from build123d import *

# Parameters (mm, degrees)
F1_DEPTH = 25.4
F2_R     = 9.525
F3_DEPTH = 6.35
F4_R     = 15.875
F5_DEPTH = 6.35
F6_R     = 9.525
F7_DEPTH = 76.2
F8_DEPTH = 6.35


with BuildPart() as f1:
    # F0 (on Top) → F1 (new body, symmetric)
    with BuildSketch(Plane.XY):
        with BuildLine():
            ThreePointArc((0, -19.05), (13.470384, -13.470384), (19.05, 0))
            ThreePointArc((19.05, 0), (13.470384, 13.470384), (0, 19.05))
            ThreePointArc((0, 19.05), (-19.05, 0), (0, -19.05))
        make_face()
    extrude(amount=F1_DEPTH, both=True)

    # F2 (on face) → F3 (cut)
    with BuildSketch(Plane.XY.offset(12.7)):
        Circle(F2_R)
    extrude(amount=-F3_DEPTH, mode=Mode.SUBTRACT)

    # F4 (on face) → F5 (cut)
    with BuildSketch(Plane.XY.offset(19.05)):
        Circle(F4_R)
    extrude(amount=-F5_DEPTH, mode=Mode.SUBTRACT)

    # F6 (on face) → F7 (cut)
    with BuildSketch(Plane.XY.offset(25.4)):
        Circle(F6_R)
    extrude(amount=-F7_DEPTH, mode=Mode.SUBTRACT)

    # F0 (on Top) → F8 (join, symmetric)
    with BuildSketch(Plane.XY):
        with BuildLine():
            ThreePointArc((0, -19.05), (-19.05, 0), (0, 19.05))
            Line((0, 19.05), (-38.1, 19.05))
            Line((-38.1, 19.05), (-38.1, -19.05))
            Line((-38.1, -19.05), (0, -19.05))
        make_face()
        with BuildLine():
            ThreePointArc((0, 19.05), (13.470384, 13.470384), (19.05, 0))
            ThreePointArc((19.05, 0), (13.470384, -13.470384), (0, -19.05))
            Line((0, -19.05), (38.1, -19.05))
            Line((38.1, -19.05), (38.1, 19.05))
            Line((38.1, 19.05), (0, 19.05))
        make_face()
    extrude(amount=F8_DEPTH, both=True)


solid = f1.part
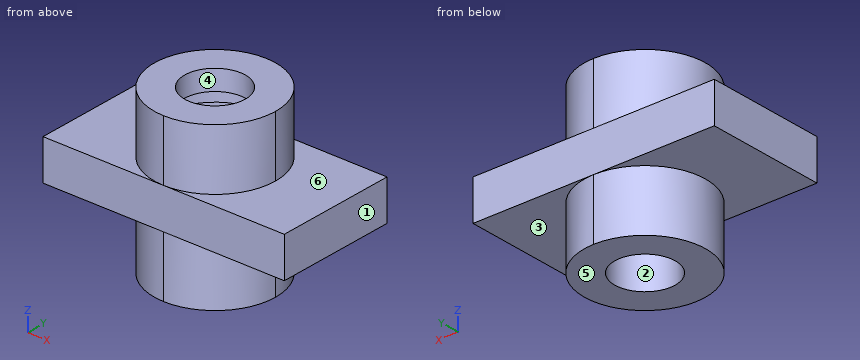
Can you work these out from the model? Positions are in its coordinate system, mm. Face numbers are marked on the shaded views. A direction names the side the tool comes from. Coordinates: 2 decimals unless noted, no trailing zeros. Order: outer loops, then holes, each group sorted by start corner. A loop starts at its lowest first (then second) coordinate and runs counter-clockwise, first axis right, second up. Notation, with made-up numbers: M 68.25,84.25 L 81.25,84.25 A29 cw 81.25,114.25 Z; hole C 14.5,-23 d7. An arc over 180 degrees is marked long. Write item = value, one per line.
(1) Suppose I cut it at C-C on x = -18. Please give me the cut outline in (y, z), plus the area to 3 significant figures.
Results are:
outline = M -19.05,-6.35 L -6.24,-6.35 L -6.24,-25.4 L 6.24,-25.4 L 6.24,-6.35 L 19.05,-6.35 L 19.05,6.35 L 6.24,6.35 L 6.24,25.4 L -6.24,25.4 L -6.24,6.35 L -19.05,6.35 Z
area = 959 mm2
(2) Suppose I cut it at A-A on y = 2.5. Please give me the cut outline in (x, z), plus the area to 3 significant figures.
Results are:
outline = M -38.1,-6.35 L -18.89,-6.35 L -18.89,-25.4 L -9.19,-25.4 L -9.19,12.7 L -15.68,12.7 L -15.68,19.05 L -9.19,19.05 L -9.19,25.4 L -18.89,25.4 L -18.89,6.35 L -38.1,6.35 Z; M 9.19,-25.4 L 18.89,-25.4 L 18.89,-6.35 L 38.1,-6.35 L 38.1,6.35 L 18.89,6.35 L 18.89,25.4 L 9.19,25.4 L 9.19,19.05 L 15.68,19.05 L 15.68,12.7 L 9.19,12.7 Z
area = 1,390 mm2
(3) Suppose I cut it at D-D on z = -9. Please give me the cut outline in (x, y) (3 decimals).
Results are:
outline = M 0,-19.05 A19.05 ccw 19.05,0 A19.05 ccw long Z; hole C 0,0 d19.05
(4) If we mould it in two halves opening along X, with no side actions, what happens to the marked faces 1, 2, 3 and 4? For each: pulls with the +X half, pulls with the -X half, needs draft (parallel to the pull), parting line crosses it, or undercut.
Results are:
face_1 = pulls with the +X half
face_2 = undercut
face_3 = needs draft
face_4 = undercut
(5) For pin 1 Ø2 at (y, z) = (11, -11) entering from +X; pin 2 Ø9.5 at (x, y) = (-3, 1.5) entering from +Z; pin 3 Ø4 at (x, z) = (15.5, -15.5) entering from +Y; pin 4 Ø1.5 at (x, y) = (-27, 1.5) entering from -Z, each with a flat end and sliding along its axis, tell me the tip position at first contact or that it passes through.
Results are:
pin_1 = 16.21
pin_2 = through
pin_3 = 13.44
pin_4 = -6.35
(6) For the marked faces 5 and 6, which set-ups out of +Z, -Z, +X, -X, +Y, -Y let a thin tool reach every point of the face, with its end or its side?
Results are:
face_5 = -Z, +X, -X, +Y, -Y
face_6 = +Z, +X
(7) I need wall thicknesses on line 1 along Y through (x, z) = (0, 15) (3 decimals); line 2 along Z through (x, y) = (-7.5, -11.5); line 3 along Z through (x, y) = (-29, 7). Which ranges of each line are inside material? Lowest first, please. Write a range as [from, to].
Results are:
line_1 = [-19.05, -15.875], [15.875, 19.05]
line_2 = [-25.4, 12.7], [19.05, 25.4]
line_3 = [-6.35, 6.35]
(8) Suppose I cut it at B-B on x = -3. Please give me the cut outline in (y, z), plus the area to 3 significant figures.
Results are:
outline = M -19.05,-6.35 L -18.81,-6.35 L -18.81,-25.4 L -9.04,-25.4 L -9.04,12.7 L -15.59,12.7 L -15.59,19.05 L -9.04,19.05 L -9.04,25.4 L -18.81,25.4 L -18.81,6.35 L -19.05,6.35 Z; M 9.04,-25.4 L 18.81,-25.4 L 18.81,-6.35 L 19.05,-6.35 L 19.05,6.35 L 18.81,6.35 L 18.81,25.4 L 9.04,25.4 L 9.04,19.05 L 15.59,19.05 L 15.59,12.7 L 9.04,12.7 Z
area = 916 mm2
